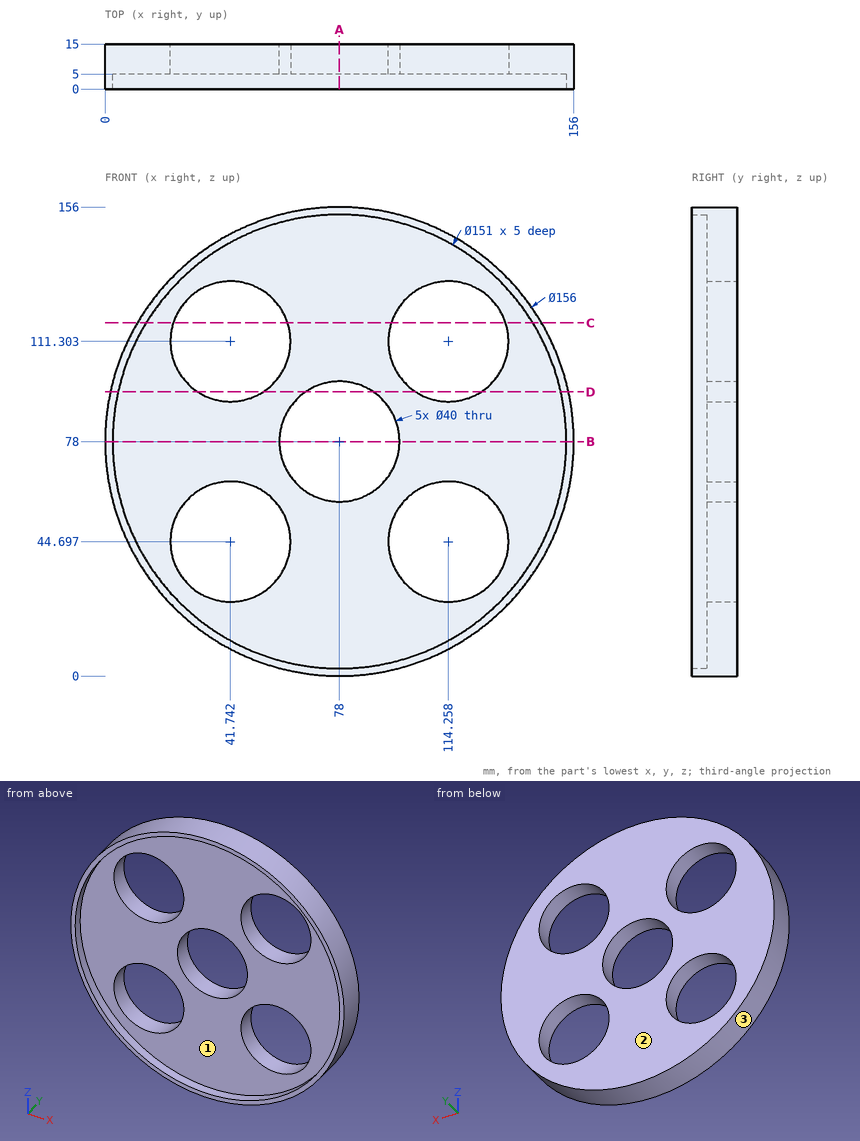
Here's the drawing with two shaded views (mm, measured from the low corner). I have some questions. Give positions to 0.01 mm unless a question says otherwise; leave off trailing zeros. Loops run counter-clockwise (first coordinate to the right, second up) from the corner with the lowest first, then second, coordinate; pieces in that order, holes last. Notation, with made-up numbers: M 1,7 L 23,7 A15 cw 23,19 Z; hole C -5.75,78.5 d9. An arc over 180 degrees is marked long. Answer in a Markdown table with one row per item.
1. Suppose I cut it at D-D on z = 94.5. Write out the boundary of the cut face in (x, y) (1 decimal).
Taken from the geometry:
| item | result |
|---|---|
| outline | M 1.8,0 L 4.3,0 L 4.3,5 L 30.9,5 L 30.9,15 L 1.8,15 Z; M 52.6,5 L 66.7,5 L 66.7,15 L 52.6,15 Z; M 89.3,5 L 103.4,5 L 103.4,15 L 89.3,15 Z; M 125.1,5 L 151.7,5 L 151.7,0 L 154.2,0 L 154.2,15 L 125.1,15 Z |
2. Suppose I cut it at A-A on x = 78. Write out the boundary of the cut face in (y, z).
Taken from the geometry:
| item | result |
|---|---|
| outline | M 0,0 L 15,0 L 15,58 L 5,58 L 5,2.5 L 0,2.5 Z; M 0,153.5 L 5,153.5 L 5,98 L 15,98 L 15,156 L 0,156 Z |
3. Suppose I cut it at C-C on z = 117.5. Write out the boundary of the cut face in (x, y), plus the area to 3 significant figures.
Taken from the geometry:
| item | result |
|---|---|
| outline | M 10.74,0 L 13.66,0 L 13.66,5 L 22.73,5 L 22.73,15 L 10.74,15 Z; M 60.76,5 L 95.24,5 L 95.24,15 L 60.76,15 Z; M 133.27,5 L 142.34,5 L 142.34,0 L 145.26,0 L 145.26,15 L 133.27,15 Z |
| area | 614 mm² |
4. Suppose I cut it at B-B on z = 78. Write out the boundary of the cut face in (x, y), plus the area to 4 significant figures.
Taken from the geometry:
| item | result |
|---|---|
| outline | M 0,0 L 2.5,0 L 2.5,5 L 58,5 L 58,15 L 0,15 Z; M 98,5 L 153.5,5 L 153.5,0 L 156,0 L 156,15 L 98,15 Z |
| area | 1,185 mm² |
5. For pin 1 Ø1.5 at (x, z) = (17, 94) entering from -Y; pin 2 Ø5 at (x, y) = (113.5, 6.5) entering from +Z (1 decimal); pin 3 Ø4 at (y, z) = (9, 36.5) entering from +X; pin 4 Ø1 at (x, z) = (43.5, 92) entering from -Y, each with a flat end and sliding along its axis, tell me the tip position at first contact or that it passes through.
Taken from the geometry:
| item | result |
|---|---|
| pin 1 | stops at y = 5 |
| pin 2 | stops at z = 148.7 |
| pin 3 | stops at x = 145.26 |
| pin 4 | passes through |
6. Thinking about a two-plate mould opening in X: for the marked faces 1, 2 and 3, which applies, released by +X, released by -X, zero draft, split by the parting line, or undercut?
Taken from the geometry:
| item | result |
|---|---|
| face 1 | undercut |
| face 2 | zero draft |
| face 3 | split by the parting line |
7. If I drill on line 1 along Z through (x, y) = (78, 2.45); line 2 along X through (y, z) = (6.25, 108.5) (1 decimal); line 3 along Z through (x, y) = (43, 13.75) (1 decimal), over which ranges is the centre line in solid material (lowest first)?
Taken from the geometry:
| item | result |
|---|---|
| line 1 | z = 0 to 2.5, 153.5 to 156 |
| line 2 | x = 6.2 to 21.9, 61.5 to 94.5, 134.1 to 149.8 |
| line 3 | z = 8.3 to 24.7, 64.7 to 91.3, 131.3 to 147.7 |
